For this review, take the finished solid that the model builds, in its own axes (mm). A direction names the side the tool comes from. Round coordinates to 2 decimals unless told otherwise and drop trailing zeros. Loops run counter-clockwise (first coordinate to the right, second up) from the corner with the lowest first, then second, coordinate; pieces in that order, holes last.
```python
from build123d import *

# Parameters (mm, degrees)
SKETCH1_W      = 18
SKETCH1_H      = 39.5
EXTRUDE1_DEPTH = 8
SKETCH4_W      = 10
SKETCH4_H      = 17.5
EXTRUDE3_DEPTH = 4
EXTRUDE4_DEPTH = 19
SKETCH4_4_R    = 1.5
EXTRUDE5_DEPTH = 9
FILLET1_R      = 2
SKETCH8_R      = 1.5
EXTRUDE6_DEPTH = 5
SKETCH9_R      = 3.5
EXTRUDE7_DEPTH = 3
FILLET2_R      = 2


with BuildPart() as part:
    # Sketch1 → Extrude1 (new body)
    with BuildSketch(Plane(origin=(0, 0, 0), x_dir=(1, 0, 0), z_dir=(0, 1, 0))):
        with Locations((0, -8.25)):
            Rectangle(SKETCH1_W, SKETCH1_H)
    extrude(amount=EXTRUDE1_DEPTH)

    # Sketch4 → Extrude3 (cut)
    with BuildSketch(Plane(origin=(0, 8, 0), x_dir=(-1, 0, 0), z_dir=(0, 1, 0))):
        with Locations((0, 19.25)):
            Rectangle(SKETCH4_W, SKETCH4_H)
    extrude(amount=-EXTRUDE3_DEPTH, mode=Mode.SUBTRACT)

    # Sketch7 → Extrude4 (cut, through all)
    with BuildSketch(Plane(origin=(9, 0, 0), x_dir=(0, 0, -1), z_dir=(1, 0, 0))):
        Polygon((-28, 4), (-10.5, 8), (-28, 8), align=None)
    extrude(amount=-EXTRUDE4_DEPTH, mode=Mode.SUBTRACT)

    # Sketch4<4> → Extrude5 (cut, through all)
    with BuildSketch(Plane(origin=(0, 8, 0), x_dir=(-1, 0, 0), z_dir=(0, 1, 0))):
        with Locations((0, 6)):
            Circle(SKETCH4_4_R)
        with Locations((0, -7)):
            Circle(SKETCH4_4_R)
    extrude(amount=-EXTRUDE5_DEPTH, mode=Mode.SUBTRACT)

    # Fillet1
    fillet1_edges = [part.edges().sort_by_distance(p)[0] for p in [
        (9, 2, 28),
        (-9, 2, 28),
    ]]
    fillet(fillet1_edges, radius=FILLET1_R)

    # Sketch8 → Extrude6 (cut, through all)
    with BuildSketch(Plane(origin=(0, 4, 0), x_dir=(-1, 0, 0), z_dir=(0, 1, 0))):
        with Locations((0, 15)):
            Circle(SKETCH8_R)
        with Locations((0, 23.5)):
            Circle(SKETCH8_R)
    extrude(amount=-EXTRUDE6_DEPTH, mode=Mode.SUBTRACT)

    # Sketch9 → Extrude7 (cut)
    with BuildSketch(Plane.XZ):
        with Locations((0, 6)):
            Circle(SKETCH9_R)
    extrude(amount=-EXTRUDE7_DEPTH, mode=Mode.SUBTRACT)

    # Fillet2
    fillet2_edges = [part.edges().sort_by_distance(p)[0] for p in [
        (-9, 4, -11.5),
        (9, 4, -11.5),
    ]]
    fillet(fillet2_edges, radius=FILLET2_R)


solid = part.part
```
(1) For faces 1 (the flat face through (-5, 5, 15)), 2 (the cylindrical face through (8.4, 2.26, 27.43)), 3 (the cylindrical face through (-0.759, 1.479, 2.583)), list the 3-axis set-ups (+Z, -Z, +X, -X, +Y, -Y) from which the entire face can be reached by the end or side of a thin tool; tool diameter is ignored.
(2) Insertion check: pin 1 Ø3 at (x, z) = (0, 20) entering from +Y; pin 2 Ø3 at (x, y) = (0, 7) entering from +Z; pin 3 Ø5 at (x, z) = (0, 6) entering from -Y. Each pin has a flat end and moves straight along its axis. Give the tip position at first contact, or say it passes through.
(3) Add section C-C (y = 5.25). Give the boundary of the cut face in (x, z).
(4) Add section A-A (z = 6). Give the boundary of the cut face in (x, y).
(5) For L1, parallel to X at y = 6.25, z = 16; L2, parallel to Y at x = -0.5, z = 7.5; L3, parallel to X at y = 5, z = 7, list the stretches that pass through material, from the lowest coordinate up.
(6) Add section B-B (x = 0). Give the boundary of the cut face in (y, z), plus the area to 3 significant figures.
(7) Add section D-D (z = -7). Give the boundary of the cut face in (x, y), plus the area to 3 significant figures.
Outcome:
1. face 1: +Z, +Y
1. face 2: +Z, +X, +Y, -Y
1. face 3: -Y
2. pin 1: stops at y = 4
2. pin 2: stops at z = 10.5
2. pin 3: stops at y = 3
3. outline: (-9, -9.5) arc R2 ccw to (-7, -11.5) - (7, -11.5) arc R2 ccw to (9, -9.5) - (9, 22.53) - (5, 22.53) - (5, 10.5) - (-5, 10.5) - (-5, 22.53) - (-9, 22.53) - close; hole circle Ø3 at (0, -7); hole circle Ø3 at (0, 6)
4. outline: (-9, 0) - (-3.5, 0) - (-3.5, 3) - (-1.5, 3) - (-1.5, 8) - (-9, 8) - close; (1.5, 3) - (3.5, 3) - (3.5, 0) - (9, 0) - (9, 8) - (1.5, 8) - close
5. L1: x = -9 to -5, 5 to 9
5. L2: y = 3 to 8
5. L3: x = -9 to -1.12, 1.12 to 9
6. outline: (0, -11.5) - (8, -11.5) - (8, -8.5) - (0, -8.5) - close; (0, -5.5) - (8, -5.5) - (8, 4.5) - (3, 4.5) - (3, 2.5) - (0, 2.5) - close; (0, 9.5) - (3, 9.5) - (3, 7.5) - (8, 7.5) - (8, 10.5) - (4, 10.5) - (4, 13.5) - (0, 13.5) - close; (0, 16.5) - (4, 16.5) - (4, 22) - (0, 22) - close; (0, 25) - (4, 25) - (4, 28) - (0, 28) - close
6. area: 162 mm2
7. outline: (-9, 0) - (-1.5, 0) - (-1.5, 8) - (-9, 8) - close; (1.5, 0) - (9, 0) - (9, 8) - (1.5, 8) - close
7. area: 120 mm2
